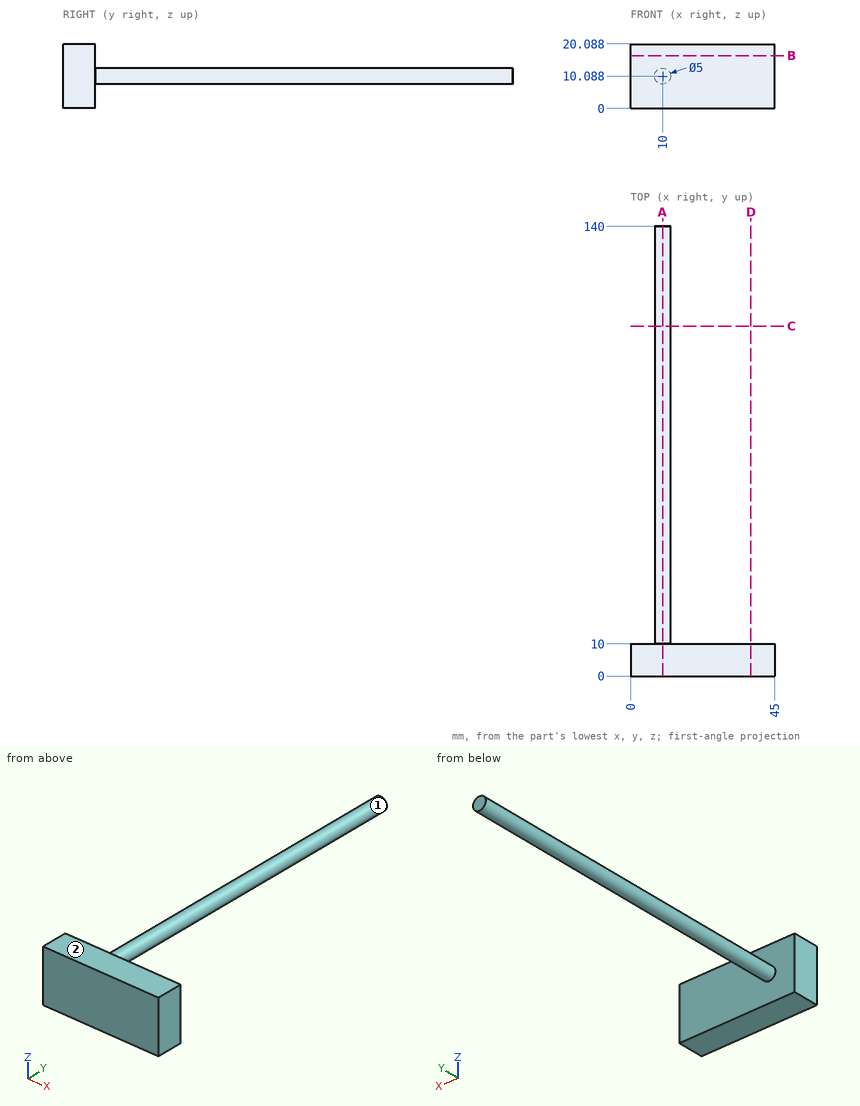
Answer from the drawing. Dimensions are ordinates in mm from the lowest x, y and z of the part. A direction names the side the tool comes from. Give positions to 0.01 mm unless a question says otherwise; leave off trailing zeros. Loops run counter-clockwise (first coordinate to the right, second up) from the corner with the lowest first, then second, coordinate; pieces in that order, holes last. Notation, with made-up numbers: (20.25, -12) - (59.25, -12) arc R33 cw to (59.25, 23) - close; hole circle Ø11 at (87.5, -5). An arc over 180 degrees is marked (long way). Answer as CSV lines item,"result". Start each with the question number.
Item 1: A cutting plane is placed at C-C on y = 109. Determine the outline of the cut face in (x, z).
Item 2: A cutting plane is placed at D-D on x = 37.5. Determine the outline of the cut face in (y, z).
Item 3: Each of these flat-tipped pins is pushed along its axis until it touches: pin 1 (8 mm diameter, centred on y = 115, z = 5, fed in from +X); pin 2 (12 mm diameter, centred on x = 18, z = 18, fed in from +Y); pin 3 (3 mm diameter, centred on x = 4.5, y = 30, fed in from +Z). Where does it stop, or does it pass through?
Item 4: A cutting plane is placed at A-A on x = 10. Determine the outline of the cut face in (y, z), then the cut area to 3 significant figures.
Item 5: For the marked faces 1 and 2, determine the directions among +Z, -Z, +X, -X, +Y, -Y from which every point of the face is accessible in a straight line to the end or side of a thin tool.
Item 6: Find the intervals of material crossed by line 1 (Y direction, x = 25, z = 5); line 2 (X direction, y = 62, z = 11.75) (1 decimal); line 3 (X direction, y = 113, z = 9), in increasing order. Write a range as from..to.
Item 7: A cutting plane is placed at B-B on z = 16.5. Determine the outline of the cut face in (x, y).
Found:
1,outline,"circle Ø5 at (10, 10.09)"
2,outline,"(0, 0) - (10, 0) - (10, 20.09) - (0, 20.09) - close"
3,pin 1,"stops at x = 12.25"
3,pin 2,"stops at y = 10"
3,pin 3,"passes through"
4,outline,"(0, 0) - (10, 0) - (10, 7.59) - (140, 7.59) - (140, 12.59) - (10, 12.59) - (10, 20.09) - (0, 20.09) - close"
4,area,"851 mm^2"
5,face 1,"+Y"
5,face 2,"+Z, +X, -X, +Y, -Y"
6,line 1,"y = 0..10"
6,line 2,"x = 8.1..11.9"
6,line 3,"x = 7.75..12.25"
7,outline,"(0, 0) - (45, 0) - (45, 10) - (0, 10) - close"
